Autodesk Inventor part; units mm, degrees
ref_plane "YZ Plane" through (0, 0, 0) normal (1, 0, 0) x (0, 1, 0)
ref_plane "XZ Plane" through (0, 0, 0) normal (0, 1, 0) x (-1, 0, 0)
ref_plane "XY Plane" through (0, 0, 0) normal (0, 0, 1) x (1, 0, 0)
sketch "Sketch1" plane through (0, 0, 0) normal (0, 0, 1) x (1, 0, 0)
  line L0 (20.32, -25.4) -> (-20.32, -25.4)
  line L1 (-20.32, -25.4) -> (-20.32, 25.4)
  line L2 (-20.32, 25.4) -> (20.32, 25.4)
  line L3 (20.32, 25.4) -> (20.32, -25.4)
  line L4 (20.32, -25.4) -> (-20.32, 25.4) construction
  line L5 (-20.32, -25.4) -> (20.32, 25.4) construction
  line L6 (15.24, -9.017) -> (-15.24, -9.017)
  line L7 (-15.24, -9.017) -> (-15.24, 9.017)
  line L8 (-15.24, 9.017) -> (15.24, 9.017)
  line L9 (15.24, 9.017) -> (15.24, -9.017)
  line L10 (15.24, -9.017) -> (-15.24, 9.017) construction
  line L11 (-15.24, -9.017) -> (15.24, 9.017) construction
  point P0 (0, 0)
  point P1 (0, 0)
  point P2 (0, 0)
  point P3 (0, 0)
  point P4 (0, 0)
  dimension "d0" = 40.64
  dimension "d1" = 30.48
  dimension "d3" = 50.8
  dimension "d4" = 18.034
extrude "Extrusion1" add sketch "Sketch1" along normal blind 6.35
sketch "Sketch2" plane through (0, 0, 6.35) normal (0, 0, 1) x (1, 0, 0)
  circle A0 centre (-14.2875, -19.3675) radius 2.2225
  circle A1 centre (14.2875, -19.3675) radius 2.2225
  line L0 (-20.32, -25.4) -> (20.32, -25.4)
  line L1 (-15.24, -9.017) -> (-15.24, 9.017)
  line L2 (-15.24, 9.017) -> (15.24, 9.017)
  line L3 (15.24, 9.017) -> (15.24, -9.017)
  line L4 (15.24, -9.017) -> (-15.24, -9.017)
  line L5 (-20.32, -25.4) -> (20.32, -25.4)
  line L6 (20.32, -25.4) -> (20.32, 25.4)
  line L7 (20.32, 25.4) -> (-20.32, 25.4)
  line L8 (-20.32, 25.4) -> (-20.32, -25.4)
  circle A2 centre (-14.2875, 19.3675) radius 2.2225
  circle A3 centre (14.2875, 19.3675) radius 2.2225
  point P0 (0, 0)
  dimension "d7" = 4.445
  dimension "d8" = 3.81
  dimension "d10" = 3.81
  dimension "d11" = 3.81
  dimension "d18" = 3.81
extrude "Extrusion2" cut sketch "Sketch2" against normal through all contours A0 | A1 | A2 | A3
fillet "Fillet1" radius 3.175 4 edges at (-20.32, 0, 6.35) (0, 25.4, 6.35) (20.32, 0, 6.35) (0, -25.4, 6.35)
chamfer "Chamfer1" distance 0.635 angle 45 4 edges at (-15.24, 0, 6.35) (0, 9.017, 6.35) (15.24, 0, 6.35) (0, -9.017, 6.35)
equation "\"d10\" = d11"
equation "\"d11\" = d8"
equation "\"d18\" = d8"
properties part number "Molex Mount"
For this review, take the finished solid that the model builds, in its own axes (mm). A direction names the side the tool comes from. Give positions to 0.01 mm unless a question says otherwise; leave off trailing zeros. Loops run counter-clockwise (first coordinate to the right, second up) from the corner with the lowest first, then second, coordinate; pieces in that order, holes last. Notation, with made-up numbers: M 86.25,67 L 142.25,67 A21 ccw 142.25,76 Z; hole C -29.5,38 d2. An arc over 180 degrees is marked long. Answer as a JSON object with one key per item and string values. Group by question number.
Q1. Tool access review of faces 4 (the flat face through (0, -9.017, 3)), 5 (the flat face through (0, 25.4, 2)): name each direction out of +Z, -Z, +X, -X, +Y, -Y from which nothing blocks a thin tool from reaching the whole face with its end or side.
Q2. Add section B-B on y = -8. Give the boundary of the cut face in (x, z) (3 decimals), and give its area (3 significant figures).
Q3. Mouldability with a two-part tool opening along Y and no side actions: class faces 1 (the cylindrical face through (-19.41, 0.36, 5.4)), 2 (the flat face through (0, -25.4, 2)), 3 (the cylindrical face through (-12.234, -20.219, 3.219)) as +Y half, -Y half, draft (parallel to the pull), parting line (faces both ways), or undercut.
Q4. Insertion check: P1, Ø3, axis at y = -4.5, z = 4, coming from the +X side; P2, Ø3.5, axis at x = 14.29, y = -19.37, coming from the -Z side; P3, Ø2, axis at x = 10, z = 4.5, coming from the +Y side; P4, Ø1, axis at x = 8.5, z = 4.5, coming from the +Y side. Each pin has a flat end and moves straight along its axis. Give the tip position at first contact, or say it passes through.
Q5. Add section A-A on x = 9. Give the boundary of the cut face in (y, z) (3 decimals).
Q6. Add section C-C on y = 21. Give the boundary of the cut face in (x, z) (3 decimals).
Q7. For probe 1 along Y at (x, z) = (-5, 2); probe 2 along Y at (x, z) = (12.5, 6); probe 3 along X at (y, z) = (-21, 1), list the stretches that pass through material, from the lowest coordinate up. Write a range as [from, to].
Q8. Add section D-D on z = 4.5. Give the boundary of the cut face in (x, y) (1 decimal).
Checked values:
{
 "1": {"face 4": "+Z, -Z", "face 5": "+Z, -Z, +X, -X, +Y"},
 "2": {"outline": "M -20.32,0 L -15.24,0 L -15.24,5.715 L -15.875,6.35 L -17.145,6.35 A3.175 ccw -20.32,3.175 Z; M 15.24,0 L 20.32,0 L 20.32,3.175 A3.175 ccw 17.145,6.35 L 15.875,6.35 L 15.24,5.715 Z", "area": "59.8 mm²"},
 "3": {"face 1": "draft", "face 2": "-Y half", "face 3": "undercut"},
 "4": {"P1": "x = 20.32", "P2": "through", "P3": "y = 25.38", "P4": "y = 25.29"},
 "5": {"outline": "M -25.4,0 L -9.017,0 L -9.017,5.715 L -9.652,6.35 L -22.225,6.35 A3.175 ccw -25.4,3.175 Z; M 9.017,0 L 25.4,0 L 25.4,3.175 A3.175 ccw 22.225,6.35 L 9.652,6.35 L 9.017,5.715 Z"},
 "6": {"outline": "M -20.32,0 L -15.796,0 L -15.796,6.35 L -17.145,6.35 A3.175 ccw -20.32,3.175 Z; M -12.779,0 L 12.779,0 L 12.779,6.35 L -12.779,6.35 Z; M 15.796,0 L 20.32,0 L 20.32,3.175 A3.175 ccw 17.145,6.35 L 15.796,6.35 Z"},
 "7": {"probe 1": "[-25.4, -9.02], [9.02, 25.4]", "probe 2": "[-23.67, -20.69], [-18.05, -9.3], [9.3, 18.05], [20.69, 23.67]", "probe 3": "[-20.32, -15.8], [-12.78, 12.78], [15.8, 20.32]"},
 "8": {"outline": "M -20,-25.1 L 20,-25.1 L 20,25.1 L -20,25.1 Z; hole C -14.3,-19.4 d4.4; hole C -14.3,19.4 d4.4; hole M -15.2,-9 L 15.2,-9 L 15.2,9 L -15.2,9 Z; hole C 14.3,-19.4 d4.4; hole C 14.3,19.4 d4.4"}
}
